Build history of the part. All positions in model axes, mm. A direction names the side the tool comes from. Give positions to 0.01 mm unless a question says otherwise; leave off trailing zeros. Loops run counter-clockwise (first coordinate to the right, second up) from the corner with the lowest first, then second, coordinate; pieces in that order, holes last. Notation, with made-up numbers: (-16, 48.25) -> (37, 48.25) arc R18 ccw to (37, 63.25) -> close; hole circle Ø10 at (-4.5, 70). An arc over 180 degrees is marked (long way). Answer as a JSON object with one key per item and string values. Group by question number.
Q1. Band-saw the part on B-B, the plane y = 0. Write the cut outline in (x, z) (3 decimals), plus the area to 3 significant figures.
Q2. Band-saw the part on D-D, the plane x = -4. Write the cut outline in (y, z), plus the area to 3 significant figures.
Q3. Wall check: probe 1 along Y at (x, z) = (-3, 4.25); probe 2 along Y at (x, z) = (2.25, 6.25); probe 3 along Y at (x, z) = (9.5, 2.75). Give the ranges that are in metal, low to high. Write a range as from..to.
Q4. Drop flat-ended pins along their axis: pin 1 (1.5 mm diameter, centred on y = -9, z = 2, fed in from +X); pin 2 (5.5 mm diameter, centred on x = 9.5, y = 0, fed in from -Z); pin 3 (0.5 mm diameter, centred on x = -2, z = 2, fed in from -Y); pin 4 (4.5 mm diameter, centred on x = -9.5, y = 0, fed in from +Z). Give the stop position or say it passes through.
Q5. Tool access for faces 1 (the flat face through (-2, 23.406, 3)), 2 (the flat face through (11.4, 0, 3.302)), 3 (the cylindrical face through (0.59, -13.87, 3.13)), 4 (the flat face through (1.588, 19, 3)): list every direction of +Z, -Z, +X, -X, +Y, -Y with a clear straight run to the whole face (end or side of a thin tool).
Q6. Two-plate mould, pull along X, no slides. Class faces 5 (the flat face through (0, 8, 6.35)), 6 (the flat face through (-1.61, 25.91, 3.22)), 7 (the cylindrical face through (-11.2, -0.1, 1.6)): pulls with the +X half, pulls with the -X half, needs draft (parallel to the pull), parting line crosses it, or undercut.
Q7. Band-saw the part on A-A, the plane z = 5.5. Write the cut outline in (x, y) (1 decimal), plus the area to 3 significant figures.
Q8. Band-saw the part on C-C, the plane x = 2. Write the cut outline in (y, z), plus the area to 3 significant figures.
Autodesk Inventor part; units mm, degrees
ref_plane "YZ Plane" through (0, 0, 0) normal (1, 0, 0) x (0, 1, 0)
ref_plane "XZ Plane" through (0, 0, 0) normal (0, 1, 0) x (-1, 0, 0)
ref_plane "XY Plane" through (0, 0, 0) normal (0, 0, 1) x (1, 0, 0)
sketch "Sketch1" plane through (0, 0, 0) normal (0, 0, 1) x (1, 0, 0)
  circle A0 centre (0, 0) radius 13.8811
  circle A1 centre (0, 0) radius 4.445
  circle A2 centre (-9.4996, 0) radius 1.7018
  circle A3 centre (9.4996, 0) radius 1.7018
  dimension "d0" = 27.7622
  dimension "d1" = 8.89
  dimension "d2" = 18.9992
  dimension "d3" = 9.4996
  dimension "d4" = 3.4036
  dimension "d5" = 3.4036
extrude "Extrusion1" add sketch "Sketch1" along normal blind 6.35
sketch "Sketch2" plane through (0, 0, 6.35) normal (0, 0, 1) x (1, 0, 0)
  line L0 (-1.5875, 4.445) -> (1.5875, 4.445)
  line L1 (1.5875, 4.445) -> (1.5875, 23.4061)
  line L2 (1.5875, 23.4061) -> (-1.5875, 23.4061)
  line L3 (-1.5875, 23.4061) -> (-1.5875, 4.445)
  circle A0 centre (0, 0) radius 4.445
  circle A1 centre (0, 0) radius 13.8811
  line L4 (0, 23.4061) -> (-3.175, 23.4061)
  line L5 (-3.175, 23.4061) -> (0, 28.4861)
  line L6 (0, 23.4061) -> (0, 21.3049) construction
  line L7 (0, 23.4061) -> (3.175, 23.4061)
  line L8 (3.175, 23.4061) -> (0, 28.4861)
  point P0 (0, 4.445)
  dimension "d8" = 3.175
  dimension "d9" = 9.525
  dimension "d10" = 5.08
  dimension "d11" = 3.175
extrude "Extrusion2" add sketch "Sketch2" against normal up to surface (6.35 mm away) contours L3 A1 L1 L0 | L3 L2 L1 A1 | L4 L5 L8 L7 L2 picked at (-1.0583, 7.56)
sketch "Sketch3" plane through (0, 0, 6.35) normal (0, 0, 1) x (1, 0, 0)
  circle A0 centre (-9.4996, 0) radius 1.7018
  circle A1 centre (-9.4996, 0) radius 2.921
  circle A2 centre (9.4996, 0) radius 1.7018
  circle A3 centre (9.4996, 0) radius 2.921
  point P0 (0, 0)
  dimension "d14" = 5.842
  dimension "d15" = 5.842
extrude "Extrusion3" cut sketch "Sketch3" against normal blind 3.048
equation "\"d15\" = d14"
properties part number "Brushless_Motor_Base_Arrow"
Worked answers:
{
 "1": {"outline": "(-13.881, 0) -> (-11.201, 0) -> (-11.201, 3.302) -> (-12.421, 3.302) -> (-12.421, 6.35) -> (-13.881, 6.35) -> close; (-7.798, 0) -> (-4.445, 0) -> (-4.445, 6.35) -> (-6.579, 6.35) -> (-6.579, 3.302) -> (-7.798, 3.302) -> close; (4.445, 0) -> (7.798, 0) -> (7.798, 3.302) -> (6.579, 3.302) -> (6.579, 6.35) -> (4.445, 6.35) -> close; (11.201, 0) -> (13.881, 0) -> (13.881, 6.35) -> (12.421, 6.35) -> (12.421, 3.302) -> (11.201, 3.302) -> close", "area": "61.7 mm2"},
 "2": {"outline": "(-13.29, 0) -> (-1.94, 0) -> (-1.94, 6.35) -> (-13.29, 6.35) -> close; (1.94, 0) -> (13.29, 0) -> (13.29, 6.35) -> (1.94, 6.35) -> close", "area": "144 mm2"},
 "3": {"probe 1": "-13.55..-3.28, 3.28..13.55, 23.41..23.69", "probe 2": "-13.7..-3.83, 3.83..13.7, 23.41..24.89", "probe 3": "-10.12..-1.7, 1.7..10.12"},
 "4": {"pin 1": "x = 11.16", "pin 2": "z = 0", "pin 3": "y = -13.77", "pin 4": "z = 3.3"},
 "5": {"face 1": "+Z, -Z, -X", "face 2": "+Z", "face 3": "+Z, -Z", "face 4": "+Z, -Z, +X"},
 "6": {"face 5": "needs draft", "face 6": "pulls with the -X half", "face 7": "undercut"},
 "7": {"outline": "(-3.2, 23.4) -> (-1.6, 23.4) -> (-1.6, 13.8) arc R13.9 ccw (long way) to (1.6, 13.8) -> (1.6, 23.4) -> (3.2, 23.4) -> (0, 28.5) -> close; hole circle Ø5.8 at (-9.5, 0); hole circle Ø8.9 at (0, 0); hole circle Ø5.8 at (9.5, 0)", "area": "536 mm2"},
 "8": {"outline": "(-13.74, 0) -> (-3.97, 0) -> (-3.97, 6.35) -> (-13.74, 6.35) -> close; (3.97, 0) -> (13.74, 0) -> (13.74, 6.35) -> (3.97, 6.35) -> close; (23.41, 0) -> (25.29, 0) -> (25.29, 6.35) -> (23.41, 6.35) -> close", "area": "136 mm2"}
}
